Design review of the part built by this model. Coordinates are the model's own, in mm. A direction names the side the tool comes from. Coordinates: 2 decimals unless noted, no trailing zeros. Loops run counter-clockwise (first coordinate to the right, second up) from the corner with the lowest first, then second, coordinate; pieces in that order, holes last. Notation, with made-up numbers: (75, -6) - (126, -6) arc R9 cw to (126, 7) - close; hole circle Ø7 at (-13, 54.5). An arc over 180 degrees is marked (long way). Use one line per item in the form item = value. Start each with the question number.
(1) Add section A-A (x = -51.5). State the section outline as (y, z) points, plus the area to 3 significant figures.
(2) Add section B-B (y = 7). State the section outline as (x, z) points.
(3) Tool access review of faces 1 (the face through (74.82, 1.97, -97.49)), 2 (the face through (98, 19, 97)): name each direction out of +Z, -Z, +X, -X, +Y, -Y from which nothing blocks a thin tool from reaching the whole face with its end or side.
(4) Add section C-C (z = -79.5). State the section outline as (x, y) points (3 decimals).
(5) The part is to be moulded in two halves that separate along X. For faces 3 (the face through (-1, 19, 101)), 4 (the face through (-105, 17, 1)), 5 (the face through (101.99, 17.24, 102.15)), say which applies: pulls with the +X half, pulls with the -X half, needs draft (parallel to the pull), parting line crosses it, or undercut.
(6) Add section D-D (x = -75). State the section outline as (y, z) points (3 decimals), plus the area to 3 significant figures.
(7) For L1, parallel to Z at x = 75, y = 3 (3 decimals); L2, parallel to X at y = 1.5, z = -92.29 (3 decimals); L3, parallel to Z at x = -76.5, y = 15.5, list the stretches that pass through material, from the lowest coordinate up.
(8) Clearance check with flat-ended pins moving along their axes: pin 1 Ø1 at (x, z) = (73.5, -57.5) entering from +Y; pin 2 Ø1.5 at (x, z) = (-100, 100) entering from +Y; pin 3 Ø1.8 at (x, y) = (-5, 16.9) entering from +Z. State where each tip first meets the part, or that it passes through.
```python
from build123d import *

# Parameters (mm, degrees)
SKETCH1_W            = 210
SKETCH1_H            = 210
BASE_DEPTH           = 4
WALLS_START          = 4
SKETCH1_3_W          = 210
SKETCH1_3_H          = 210
SKETCH1_3_W_2        = 202
SKETCH1_3_H_2        = 202
WALLS_DEPTH          = 30
SCREWMOUNTS_DEPTH    = 30
SKETCH2_5_R          = 1.5
SCREWHOLES_DEPTH     = 12.5
ROUNDEDCORNERS_R     = 10
BACKHOLEMOUNTS_DEPTH = 4
SKETCH4_R            = 1.5
SKETCH4_W            = 30
SKETCH4_H            = 10
BATTERYPACK_DEPTH    = 4


with BuildPart() as part:
    # Sketch1 → Base (new body)
    with BuildSketch(Plane(origin=(0, 0, 0), x_dir=(1, 0, 0), z_dir=(0, 1, 0))):
        Rectangle(SKETCH1_W, SKETCH1_H)
    extrude(amount=BASE_DEPTH)

    # Sketch1<3> → Walls (add)
    with BuildSketch(Plane(origin=(0, 0, 0), x_dir=(1, 0, 0), z_dir=(0, 1, 0)).offset(WALLS_START)):
        Rectangle(SKETCH1_3_W, SKETCH1_3_H)
        Rectangle(SKETCH1_3_W_2, SKETCH1_3_H_2, mode=Mode.SUBTRACT)
    extrude(amount=WALLS_DEPTH)

    # Sketch2 → ScrewMounts (add)
    with BuildSketch(Plane(origin=(0, 34, 0), x_dir=(1, 0, 0), z_dir=(0, 1, 0))):
        with BuildLine():
            Line((-101, 101), (-101, 96))
            ThreePointArc((-101, 96), (-97.464466094, 97.464466094), (-96, 101))
            Line((-96, 101), (-101, 101))
        make_face()
        with BuildLine():
            Line((-101, -101), (-96, -101))
            ThreePointArc((-96, -101), (-97.464466094, -97.464466094), (-101, -96))
            Line((-101, -96), (-101, -101))
        make_face()
        with BuildLine():
            Line((101, 101), (96, 101))
            ThreePointArc((96, 101), (97.464466094, 97.464466094), (101, 96))
            Line((101, 96), (101, 101))
        make_face()
        with BuildLine():
            Line((101, -101), (101, -96))
            ThreePointArc((101, -96), (97.464466094, -97.464466094), (96, -101))
            Line((96, -101), (101, -101))
        make_face()
    extrude(amount=-SCREWMOUNTS_DEPTH)

    # Sketch2<5> → ScrewHoles (cut)
    with BuildSketch(Plane(origin=(0, 34, 0), x_dir=(1, 0, 0), z_dir=(0, 1, 0))):
        with Locations((-99.833273811, 99.833273811)):
            Circle(SKETCH2_5_R)
        with Locations((-99.833273811, -99.833273811)):
            Circle(SKETCH2_5_R)
        with Locations((99.833273811, 99.833273811)):
            Circle(SKETCH2_5_R)
        with Locations((99.833273811, -99.833273811)):
            Circle(SKETCH2_5_R)
    extrude(amount=-SCREWHOLES_DEPTH, mode=Mode.SUBTRACT)

    # RoundedCorners
    roundedcorners_edges = [part.edges().sort_by_distance(p)[0] for p in [
        (-105, 17, 105),
        (105, 17, 105),
        (105, 17, -105),
        (-105, 17, -105),
    ]]
    fillet(roundedcorners_edges, radius=ROUNDEDCORNERS_R)

    # Sketch3 → BackHoleMounts (cut)
    with BuildSketch(Plane.XZ):
        with BuildLine():
            Line((-77.985, 80), (-77.985, 61.974012195))
            ThreePointArc((-77.985, 61.974012195), (-75, 52.505), (-72.015, 61.974012195))
            Line((-72.015, 61.974012195), (-72.015, 80))
            ThreePointArc((-72.015, 80), (-75, 82.985), (-77.985, 80))
        make_face()
        with BuildLine():
            Line((77.985, 80), (77.985, 61.974012195))
            ThreePointArc((77.985, 61.974012195), (75, 52.505), (72.015, 61.974012195))
            Line((72.015, 61.974012195), (72.015, 80))
            ThreePointArc((72.015, 80), (75, 82.985), (77.985, 80))
        make_face()
        with BuildLine():
            Line((72.015, -70), (72.015, -88.025987805))
            ThreePointArc((72.015, -88.025987805), (75, -97.495), (77.985, -88.025987805))
            Line((77.985, -88.025987805), (77.985, -70))
            ThreePointArc((77.985, -70), (75, -67.015), (72.015, -70))
        make_face()
        with BuildLine():
            Line((-77.985, -70), (-77.985, -88.025987805))
            ThreePointArc((-77.985, -88.025987805), (-75, -97.495), (-72.015, -88.025987805))
            Line((-72.015, -88.025987805), (-72.015, -70))
            ThreePointArc((-72.015, -70), (-75, -67.015), (-77.985, -70))
        make_face()
    extrude(amount=-BACKHOLEMOUNTS_DEPTH, mode=Mode.SUBTRACT)

    # Sketch4 → BatteryPack (cut)
    with BuildSketch(Plane.XY.offset(105)):
        with Locations((75, 16.9)):
            Circle(SKETCH4_R)
        with Locations((-5, 16.9)):
            Circle(SKETCH4_R)
        with Locations((-50, 16.9)):
            Rectangle(SKETCH4_W, SKETCH4_H)
    extrude(amount=-BATTERYPACK_DEPTH, mode=Mode.SUBTRACT)


solid = part.part
```
Computed values:
q1.outline = (0, -105) - (34, -105) - (34, -101) - (4, -101) - (4, 101) - (11.9, 101) - (11.9, 105) - (0, 105) - close; (21.9, 101) - (34, 101) - (34, 105) - (21.9, 105) - close
q1.area = 1,040 mm^2
q2.outline = (-105, -95) arc R10 ccw to (-95, -105) - (95, -105) arc R10 ccw to (105, -95) - (105, 95) arc R10 ccw to (95, 105) - (-95, 105) arc R10 ccw to (-105, 95) - close; hole (-101, -96) arc R5 cw to (-96, -101) - (96, -101) arc R5 cw to (101, -96) - (101, 96) arc R5 cw to (96, 101) - (-96, 101) arc R5 cw to (-101, 96) - close
q3.face_1 = +Y, -Y
q3.face_2 = +Y
q4.outline = (-105, 0) - (-77.985, 0) - (-77.985, 4) - (-101, 4) - (-101, 34) - (-105, 34) - close; (-72.015, 0) - (72.015, 0) - (72.015, 4) - (-72.015, 4) - close; (77.985, 0) - (105, 0) - (105, 34) - (101, 34) - (101, 4) - (77.985, 4) - close
q5.face_3 = undercut
q5.face_4 = pulls with the -X half
q5.face_5 = pulls with the +X half
q6.outline = (0, -105) - (34, -105) - (34, -101) - (4, -101) - (4, -97.495) - (0, -97.495) - close; (0, -67.015) - (4, -67.015) - (4, 52.505) - (0, 52.505) - close; (0, 82.985) - (4, 82.985) - (4, 101) - (34, 101) - (34, 105) - (0, 105) - close
q6.area = 836 mm^2
q7.L1 = -105 to -97.495, -67.015 to 52.505, 82.985 to 105
q7.L2 = -105 to -80.205, -69.795 to 69.795, 80.205 to 105
q7.L3 = -105 to -101, 101 to 105
q8.pin_1 = 4
q8.pin_2 = 21.5
q8.pin_3 = -101
